For this review, take the finished solid that the model builds, in its own axes (mm). Face numbers are marked on the shaded views. A direction names the side the tool comes from. Round coordinates to 2 decimals unless told otherwise and drop trailing zeros. Order: outer loops, then holes, each group sorted by start corner. A loop starts at its lowest first (then second) coordinate and runs counter-clockwise, first axis right, second up. Notation, with made-up numbers: (-2, 48.5) - (7, 48.5) arc R32 ccw to (7, 79.5) - close; hole circle Ø10 at (54.25, -25.5). An arc over 180 degrees is marked (long way). One line per question, with ' | ' between items.
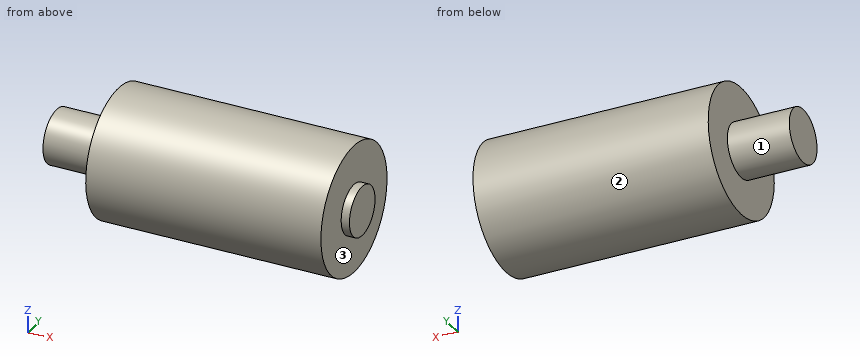
```python
from build123d import *

# Parameters (mm, degrees)
SKETCH_1_R      = 15.5
EXTRUDE_1_DEPTH = 57
SKETCH_2_R      = 6.5
EXTRUDE_2_DEPTH = 15
SKETCH_3_R      = 6
EXTRUDE_3_DEPTH = 2


with BuildPart() as part:
    # 草图1 → 凸台-拉伸1 (new body)
    with BuildSketch(Plane(origin=(0, 0, 0), x_dir=(0, 0, -1), z_dir=(1, 0, 0))):
        Circle(SKETCH_1_R)
    extrude(amount=EXTRUDE_1_DEPTH)

    # 草图2 → 凸台-拉伸2 (add)
    with BuildSketch(Plane(origin=(0, 0, 0), x_dir=(0, 0, -1), z_dir=(1, 0, 0))):
        Circle(SKETCH_2_R)
    extrude(amount=-EXTRUDE_2_DEPTH)

    # 草图3 → 凸台-拉伸3 (add)
    with BuildSketch(Plane(origin=(57, 0, 0), x_dir=(0, 0, -1), z_dir=(1, 0, 0))):
        Circle(SKETCH_3_R)
    extrude(amount=EXTRUDE_3_DEPTH)


solid = part.part
```
(1) We need section B-B on x = 52. State the section outline as (y, z) points, plus the area to 3 significant figures.
Output values:
outline: circle Ø31 at (0, 0) | area: 755 mm^2
(2) We need section A-A on z = 3.5. State the section outline as (x, y) points, plus the area to 3 significant figures.
Output values:
outline: (-15, -5.48) - (0, -5.48) - (0, -15.1) - (57, -15.1) - (57, -4.87) - (59, -4.87) - (59, 4.87) - (57, 4.87) - (57, 15.1) - (0, 15.1) - (0, 5.48) - (-15, 5.48) - close | area: 1,910 mm^2
(3) We need section D-D on x = -8.5. State the section outline as (y, z) points.
Output values:
outline: circle Ø13 at (0, 0)
(4) We need section C-C on z = 0. State the section outline as (x, y) points.
Output values:
outline: (-15, -6.5) - (0, -6.5) - (0, -15.5) - (57, -15.5) - (57, -6) - (59, -6) - (59, 6) - (57, 6) - (57, 15.5) - (0, 15.5) - (0, 6.5) - (-15, 6.5) - close
(5) For probe 1 along X at (y, z) = (-9, -5.5); probe 2 along Y at (x, z) = (-2.5, -2.5); probe 3 along Y at (x, z) = (6, -10), list the stretches that pass through material, from the lowest coordinate up. Write a range as [from, to].
Output values:
probe 1: [0, 57] | probe 2: [-6, 6] | probe 3: [-11.84, 11.84]
(6) For the marked faces 1, 2 and 3, list the 3-axis set-ups (+Z, -Z, +X, -X, +Y, -Y) from which the entire face can be reached by the end or side of a thin tool; tool diameter is ignored.
Output values:
face 1: -X | face 2: +X, -X | face 3: +X
(7) Insertion check: pin 1 (5 mm diameter, centred on x = 41, z = 6.5, fed in from +Y) (3 decimals); pin 2 (1 mm diameter, centred on y = 8, z = 0, fed in from +X); pin 3 (3 mm diameter, centred on x = 24, y = -7, fed in from -Z). Each pin has a flat end and moves straight along its axis. Give the tip position at first contact, or say it passes through.
Output values:
pin 1: y = 14.975 | pin 2: x = 57 | pin 3: z = -14.49
